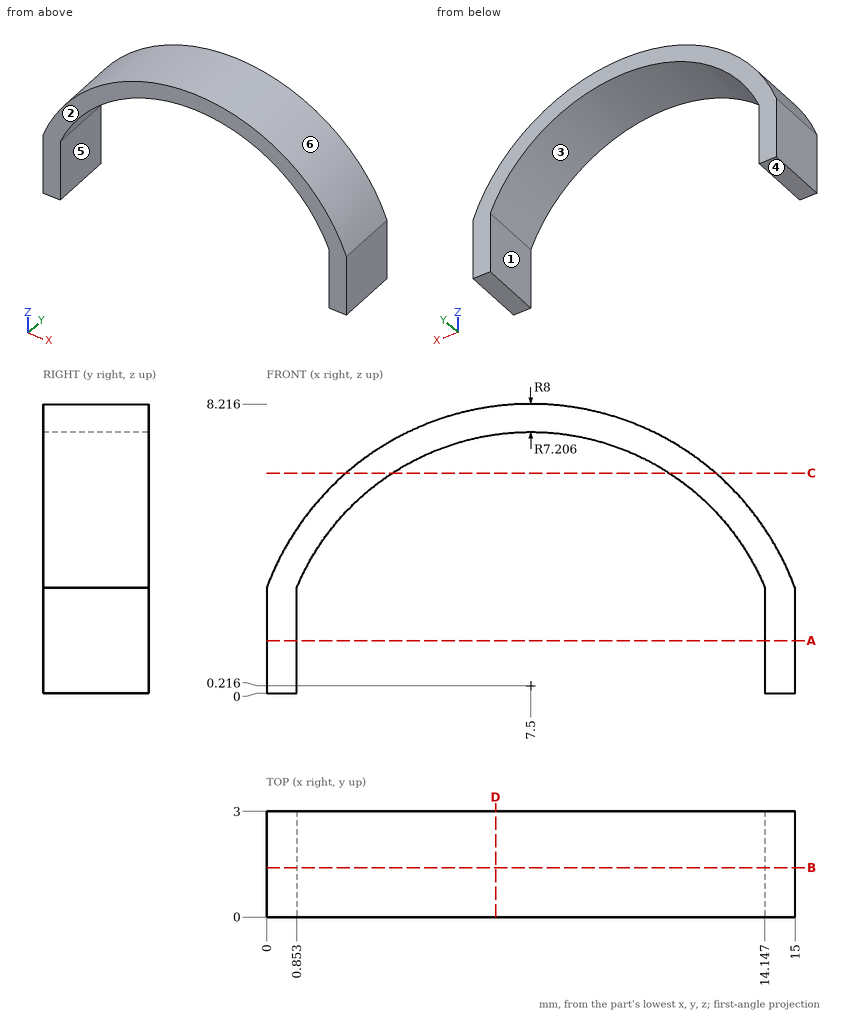
Study the drawing (mm; zero at the part's minimum x, y, z) and answer. A direction names the side the tool comes from. Round coordinates to 2 decimals unless told otherwise and drop trailing zeros. Write each loop counter-clockwise with the first axis right and the second up, starting at its lowest first coordinate (ties: lowest second). Pieces come first, ordered by that corner, then holes. Notation, with made-up numbers: (6, 37) - (52, 37) arc R18 ccw to (52, 61) - close; hole circle Ø5 at (-8, 4). An arc over 180 degrees is marked (long way). Return JSON: item names as keys, results as strings. Group by question number.
Q1. For the marked faces 1 and 2, determine the directions among +Z, -Z, +X, -X, +Y, -Y from which every point of the face is accessible in a straight line to the end or side of a thin tool.
Q2. Find the intervals of material crossed by L1, parallel to X at y = 2.6, z = 0.75; L2, parallel to X at y = 1.3, z = 3.5 (1 decimal); L3, parallel to Z at x = 8, y = 1.5 (1 decimal), in increasing order.
Q3. The part is cut by section A-A on z = 1.5. Write down the section's boundary in (x, y).
Q4. The part is cut by section B-B on y = 1.4. Write down the section's boundary in (x, z).
Q5. This flat-tipped pin is pushed along its axis until it touches: pin 1 Ø1 at (x, y) = (10.5, 2.5) entering from +Z (1 decimal). Where does it stop, or does it pass through?
Q6. The part is cut by section D-D on x = 6.5. Write down the section's boundary in (y, z).
Q7. The part is cut by section C-C on z = 6.25. Write down the section's boundary in (x, y).
Q8. The mould has two halves that part along X. Classify the marked faces 3, 4, 5 and 6: released by +X, released by -X, zero draft, split by the parting line, or undercut.
Solved:
{
 "1": {"face 1": "-Z, +Y, -Y", "face 2": "+Z, -Z, +X, -X, -Y"},
 "2": {"L1": "0 to 0.85, 14.15 to 15", "L2": "0.2 to 1.1, 13.9 to 14.8", "L3": "7.4 to 8.2"},
 "3": {"outline": "(0, 0) - (0.85, 0) - (0.85, 3) - (0, 3) - close; (14.15, 0) - (15, 0) - (15, 3) - (14.15, 3) - close"},
 "4": {"outline": "(0, 0) - (0.85, 0) - (0.85, 3) arc R7.21 cw to (14.15, 3) - (14.15, 0) - (15, 0) - (15, 3) arc R8 ccw to (0, 3) - close"},
 "5": {"pin 1": "z = 7.8"},
 "6": {"outline": "(0, 7.35) - (3, 7.35) - (3, 8.15) - (0, 8.15) - close"},
 "7": {"outline": "(2.25, 0) - (3.56, 0) - (3.56, 3) - (2.25, 3) - close; (11.44, 0) - (12.75, 0) - (12.75, 3) - (11.44, 3) - close"},
 "8": {"face 3": "undercut", "face 4": "zero draft", "face 5": "undercut", "face 6": "split by the parting line"}
}
